Drawing for the job (mm, zero at the part's lowest x, y, z). A direction names the side the tool comes from. Give positions to 0.01 mm unless a question says otherwise; leave off trailing zeros. Loops run counter-clockwise (first coordinate to the right, second up) from the corner with the lowest first, then second, coordinate; pieces in that order, holes last.
1) Wall check: line 1 (X direction, y = 10.25, z = 2); line 2 (X direction, y = 5.75, z = 9); line 3 (Z direction, x = 6.25, y = 1). Give the ranges that are in metal, low to high.
2) Flat gauge pins, fed straight in: P1, Ø2, axis at x = 8.5, z = 4.5, coming from the -Y side; P2, Ø3, axis at x = 6.5, y = 3, coming from the +Z side. Where does each tip first touch, or does it go through?
3) Band-saw the part on C-C on x = 1.75. List the corners of the cut face in (y, z), then the cut area to 3 significant figures.
4) Two-plate mould, pull along X, no slides. Class the marked faces 3, 4, 5 and 6: +X half, -X half, draft (parallel to the pull), parting line (faces both ways), or undercut.
5) Band-saw the part on B-B on y = 4. List the corners of the cut face in (x, z).
6) Band-saw the part on D-D on x = 5. List the corners of the cut face in (y, z).
7) Band-saw the part on A-A on z = 5. List the corners of the cut face in (x, y).
8) 3-axis set-ups, long thin cutter, end or side, ignore diameter. For the marked faces 1 and 2: which of +Z, -Z, +X, -X, +Y, -Y reach the whole face in a straight line?
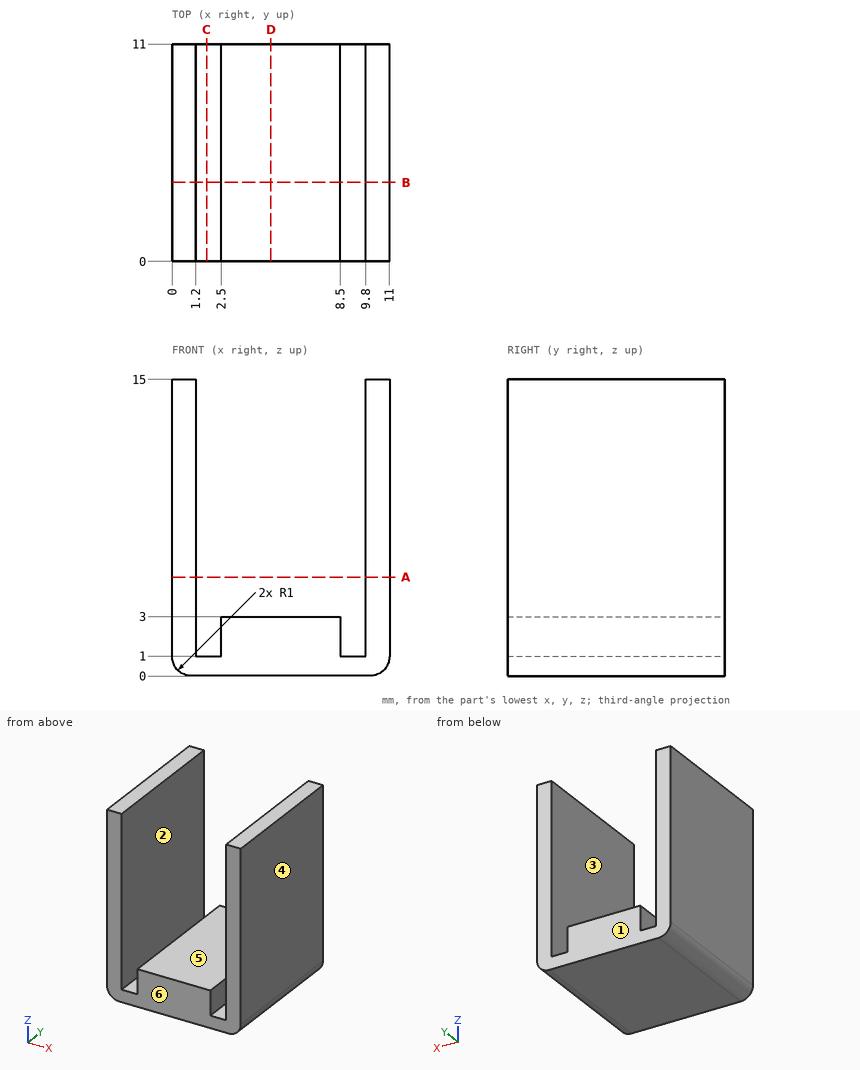
Findings below:
1. line 1: x = 0 to 1.2, 2.5 to 8.5, 9.8 to 11
1. line 2: x = 0 to 1.2, 9.8 to 11
1. line 3: z = 0 to 3
2. P1: passes through
2. P2: stops at z = 3
3. outline: (0, 0) - (11, 0) - (11, 1) - (0, 1) - close
3. area: 11.0 mm2
4. face 3: undercut
4. face 4: +X half
4. face 5: undercut
4. face 6: draft
5. outline: (0, 1) arc R1 ccw to (1, 0) - (10, 0) arc R1 ccw to (11, 1) - (11, 15) - (9.8, 15) - (9.8, 1) - (8.5, 1) - (8.5, 3) - (2.5, 3) - (2.5, 1) - (1.2, 1) - (1.2, 15) - (0, 15) - close
6. outline: (0, 0) - (11, 0) - (11, 3) - (0, 3) - close
7. outline: (0, 0) - (1.2, 0) - (1.2, 11) - (0, 11) - close; (9.8, 0) - (11, 0) - (11, 11) - (9.8, 11) - close
8. face 1: +Z, -Z, +X, -X, +Y
8. face 2: +Z, +Y, -Y
